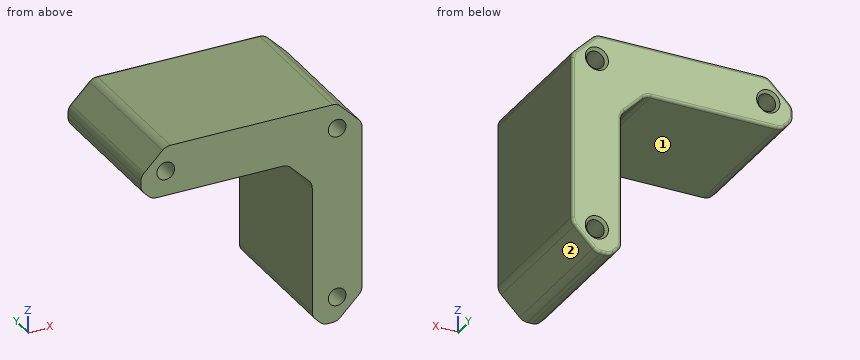
Autodesk Inventor part; units mm, degrees
ref_plane "YZ Plane" through (0, 0, 0) normal (1, 0, 0) x (0, 1, 0)
ref_plane "XZ Plane" through (0, 0, 0) normal (0, 1, 0) x (-1, 0, 0)
ref_plane "XY Plane" through (0, 0, 0) normal (0, 0, 1) x (1, 0, 0)
sketch "Sketch1" plane through (0, 0, 0) normal (0, 1, 0) x (-1, 0, 0)
  line L0 (0, 0) -> (0, -35.5002)
  line L1 (9, -9) -> (35.5, -9)
  line L2 (35.5002, 0) -> (0, 0)
  circle A0 centre (4.5, -4.5) radius 1.6
  circle A1 centre (35.5, -4.5) radius 1.6
  circle A2 centre (4.5, -35.5) radius 1.6
  line L3 (9, -35.5) -> (9, -9)
  line L4 (31, -9) -> (40, -9)
  line L5 (40, -9) -> (40, 0)
  line L6 (40, 0) -> (31, 0)
  line L7 (31, -9) -> (40, 0) construction
  line L8 (40, -9) -> (31, 0) construction
  line L9 (0, -31) -> (0, -40)
  line L10 (0, -40) -> (9, -40)
  line L11 (9, -40) -> (9, -31)
  line L12 (9, -31) -> (0, -40) construction
  line L13 (0, -31) -> (9, -40) construction
  arc A3 (35.4998, 0) -> (35.4998, 0) centre (35.5, -4.5) ccw
  point P0 (0, 0)
  point P1 (0, -9)
  dimension "d8" = 3.2
  dimension "d21" = 4.5
  dimension "d22" = 31
  dimension "d23" = 31
  dimension "d38" = 4.5
extrude "Extrusion1" add sketch "Sketch1" along normal blind 26
chamfer "Chamfer2" distance 2 angle 45 2 edges at (-40, 13, -9) (-9, 13, -40)
chamfer "Chamfer3" distance 4.5 angle 45 4 edges at (-40, 13, 0) (0, 13, 0) (0, 13, -40) (-9, 13, -9)
fillet "Fillet4" radius 2 12 edges at (-40, 13, -7) (-35.5, 13, 0) (-40, 13, -4.5) (-38, 13, -9) (-9, 13, -38) (-7, 13, -40) (-4.5, 13, -40) (0, 13, -35.5) (0, 13, -4.5) (-4.5, 13, 0) (-13.5, 13, -9) (-9, 13, -13.5)
fillet "Fillet5" radius 0.5 23 edges at (-4.5631, 26, -0.1522) (-2.25, 26, -2.25) (-0.1522, 26, -4.5631) (0, 26, -20) (-0.1522, 26, -35.4369) (-2.25, 26, -37.75) (-4.5631, 26, -39.8478) (-5.75, 26, -40) (-6.9369, 26, -39.8478) (-8, 26, -39) (-8.8478, 26, -37.9369) (-9, 26, -24.9142) (-9, 26, -36.3358) (-24.9142, 26, -9) (-36.3358, 26, -9) (-37.9369, 26, -8.8478) (-39, 26, -8) (-39.8478, 26, -6.9369) (-40, 26, -5.75) (-39.8478, 26, -4.5631) (-37.75, 26, -2.25) (-35.4369, 26, -0.1522) (-20, 26, 0)
chamfer "Chamfer4" distance 0.5 angle 45 3 edges at (-33.9, 26, -4.5) (-2.9, 26, -4.5) (-2.9, 26, -35.5)
properties part number "stepper spacer"
Model file for the job. Use its own axes, mm. Face numbers are marked on the shaded views. A direction names the side the tool comes from. Coordinates: 2 decimals unless noted, no trailing zeros. Write each loop counter-clockwise with the first axis right and the second up, starting at its lowest first coordinate (ties: lowest second). Pieces come first, ordered by that corner, then holes. Notation, with made-up numbers: (46.5, 14) - (54.5, 14) arc R23 cw to (54.5, 37) - close; hole circle Ø1 at (87.5, 71.25). An arc over 180 degrees is marked (long way). One line per item, written item: value. Start each with the question number.
1. Tool access for the marked faces 1 and 2: list every direction of +Z, -Z, +X, -X, +Y, -Y with a clear straight run to the whole face (end or side of a thin tool).
2. Flat gauge pins, fed straight in: pin 1 (6 mm diameter, centred on x = -33, y = 7, fed in from -Z); pin 2 (2 mm diameter, centred on y = 8, z = -4, fed in from +X). Where does each tip first touch, or does it go through?
3. Slice it at B-B (x = -16). Write the cut outline in (y, z), plus the area to 3 significant figures.
4. Probe line 1 (Z direction, x = -4.5, y = 14); line 2 (X direction, y = 12.5, z = -5.5); line 3 (X direction, y = 20, z = -30.5). List the from-to ranges inside material, lowest first. Write a range as from..to.
5. Slice it at A-A (z = -17.5). Write the cut outline in (x, y).
Answers below:
1. face 1: -Z, -X, +Y, -Y
1. face 2: -Z, +X, +Y, -Y
2. pin 1: stops at z = -9
2. pin 2: stops at x = -0.03
3. outline: (0, -9) - (25.5, -9) arc R0.5 ccw to (26, -8.5) - (26, -0.5) arc R0.5 ccw to (25.5, 0) - (0, 0) - close
3. area: 234 mm^2
4. line 1: z = -39.82..-37.1, -33.9..-6.1, -2.9..-0.18
4. line 2: x = -40..-36.75, -34.25..-5.75, -3.25..0
4. line 3: x = -9..0
5. outline: (-9, 0) - (0, 0) - (0, 25.5) arc R0.5 ccw to (-0.5, 26) - (-8.5, 26) arc R0.5 ccw to (-9, 25.5) - close
